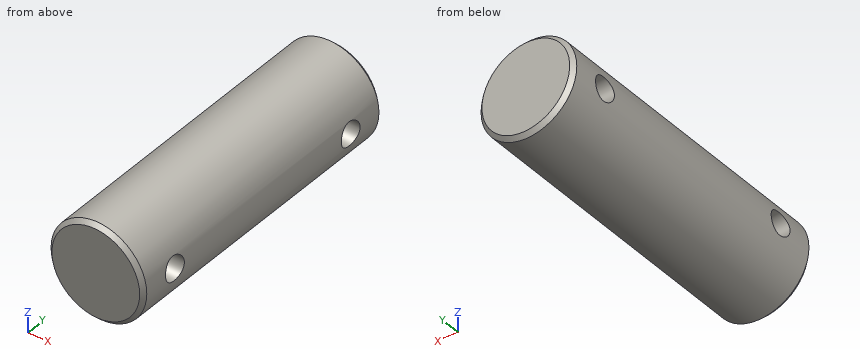
Autodesk Inventor part; units mm, degrees
ref_plane "YZ Plane" through (0, 0, 0) normal (1, 0, 0) x (0, 1, 0)
ref_plane "XZ Plane" through (0, 0, 0) normal (0, 1, 0) x (-1, 0, 0)
ref_plane "XY Plane" through (0, 0, 0) normal (0, 0, 1) x (1, 0, 0)
sketch "Sketch1" plane through (0, 0, 0) normal (0, 1, 0) x (-1, 0, 0)
  circle A0 centre (0, 0) radius 6
  dimension "d0" = 12
extrude "Extrusion1" add sketch "Sketch1" along normal blind 37
sketch "Sketch2" plane through (0, 37, 0) normal (0, 1, 0) x (1, 0, 0)
  circle A0 centre (0, 0) radius 6
  dimension "d3" = 12
extrude "Extrusion2" add sketch "Sketch2" along normal blind 0.5 draft -45
sketch "Sketch3" plane through (0, 0, 0) normal (0, -1, 0) x (1, 0, 0)
  circle A0 centre (0, 0) radius 6
  dimension "d6" = 12
extrude "Extrusion3" add sketch "Sketch3" along normal blind 0.5 draft -45
sketch "Sketch5" plane through (0, 0, 0) normal (0, 1, 0) x (-1, 0, 0)
  point P0 (0, 0)
sketch "Sketch7" plane through (0, 0, 0) normal (1, 0, 0) x (0, 1, 0)
  circle A0 centre (4.5, 0.3338) radius 1.5
  point P0 (0, 0)
  dimension "d15" = 3
extrude "Extrusion6" cut sketch "Sketch7" against normal mid plane 12
sketch "Sketch8" plane through (0, 0, 0) normal (1, 0, 0) x (0, 1, 0)
  circle A0 centre (32.5, 0) radius 1.5
  point P0 (0, 0)
  dimension "d18" = 3
extrude "Extrusion7" cut sketch "Sketch8" against normal mid plane 12
properties part number "crankshaft pin" material "Stainless Steel"
Design review of the part built by this model. Coordinates are the model's own, in mm. Give positions to 0.01 mm unless a question says otherwise; leave off trailing zeros. Write each loop counter-clockwise with the first axis right and the second up, starting at its lowest first coordinate (ties: lowest second). Pieces come first, ordered by that corner, then holes. Notation, with made-up numbers: M 63.5,4.25 L 113.5,4.25 A16 cw 113.5,20.25 Z; hole C 46.5,20.5 d4. An arc over 180 degrees is marked long. Answer as a JSON object with one key per item and string values. Group by question number.
1) We need section D-D (y = 27). Give the boundary of the cut face in (x, z), and give its area (3 significant figures).
2) Clearance check with flat-ended pins moving along their axes: pin 1 Ø1.5 at (y, z) = (33.5, -5) entering from +X; pin 2 Ø5 at (y, z) = (22, 3.5) entering from -X; pin 3 Ø1 at (y, z) = (19, -2.5) entering from +X; pin 4 Ø2.5 at (y, z) = (4.5, 0.33) entering from +X. State where each tip first meets the part, or that it passes through.
3) We need section C-C (y = 4.5). Give the boundary of the cut face in (x, z), and give its area (3 significant figures).
4) We need section B-B (x = 0). Give the boundary of the cut face in (y, z).
5) For line 1 along Z through (x, y) = (-0.25, 4.5); line 2 along Y through (x, z) = (1.5, -0.75); line 3 along Y through (x, z) = (-0.5, 0), list the stretches that pass through material, from the lowest coordinate up.
6) We need section A-A (z = 0). Give the boundary of the cut face in (x, y), and give its area (3 significant figures).
Answer key:
{
 "1": {"outline": "C 0,0 d12", "area": "113 mm²"},
 "2": {"pin 1": "stops at x = 4.24", "pin 2": "stops at x = -5.92", "pin 3": "stops at x = 5.66", "pin 4": "passes through"},
 "3": {"outline": "M -5.89,-1.17 A6 ccw 5.89,-1.17 Z; M -5.71,1.83 L 5.71,1.83 A6 ccw Z", "area": "77.5 mm²"},
 "4": {"outline": "M -0.5,-5.5 L 0,-6 L 37,-6 L 37.5,-5.5 L 37.5,5.5 L 37,6 L 0,6 L -0.5,5.5 Z; hole C 4.5,0.33 d3; hole C 32.5,0 d3"},
 "5": {"line 1": "z = -5.99 to -1.17, 1.83 to 5.99", "line 2": "y = -0.5 to 3.46, 5.54 to 31.2, 33.8 to 37.5", "line 3": "y = -0.5 to 3.04, 5.96 to 31, 34 to 37.5"},
 "6": {"outline": "M -6,0 L -5.5,-0.5 L 5.5,-0.5 L 6,0 L 6,3.04 L -6,3.04 Z; M -6,5.96 L 6,5.96 L 6,31 L -6,31 Z; M -6,34 L 6,34 L 6,37 L 5.5,37.5 L -5.5,37.5 L -6,37 Z", "area": "384 mm²"}
}
